Here's how the part is built. I have some questions about the finished solid (model axes, mm). Round coordinates to 2 decimals unless told otherwise and drop trailing zeros. Loops run counter-clockwise (first coordinate to the right, second up) from the corner with the lowest first, then second, coordinate; pieces in that order, holes last. Notation, with made-up numbers: (-39.5, -9) - (-26.5, -9) arc R36 ccw to (-26.5, 27) - close; hole circle Ø8 at (31, 19.25). An arc over 180 degrees is marked (long way). Answer as a JSON object with one key per item and string values. Group by question number.
1) I want a section at B-B, the plane y = 0.6. Give the number of separate pieces and of enclosed holes in the cut face, then the cut area to 3 significant figures.
2) Will these pins go through, and if not, where does the flat tip stop? P1, Ø0.5, axis at y = 0.5, z = 80.5, coming from the +X side; P2, Ø0.5, axis at y = 0.5, z = -101.5, coming from the -X side.
3) I want a section at D-D, the plane z = 86.5. Please give me the cut outline in (x, y), then the cut area to 3 significant figures.
4) If we mould it in two halves opening along X, with no side actions, what happens to faces 1 (the face through (41.748, 0.493, 105.846)), 2 (the face through (33.07, 0.49, 104.63)), 3 (the face through (1, 0, -2))? For each: pulls with the +X half, pulls with the -X half, needs draft (parallel to the pull), parting line crosses it, or undercut.
5) If I drill on line 1 along Z through (x, y) = (-19, 0.3); line 2 along Z through (x, y) = (12.5, 0.8); line 3 along Z through (x, y) = (26.5, 0.5), over which ranges is the centre line in solid material (lowest first)? Write a range as [from, to].
6) I want a section at C-C, the plane z = 36.5. Please give me the cut outline in (x, y).
7) I want a section at A-A, the plane x = -24. Please give me the cut outline in (y, z).
from build123d import *

# Parameters (mm, degrees)
SKETCH1_R           = 1.95
BOSS_EXTRUDE1_DEPTH = 1


with BuildPart() as part:
    # Sketch1 → Boss-Extrude1 (new body)
    with BuildSketch(Plane(origin=(0, 0, 0), x_dir=(1, 0, 0), z_dir=(0, 1, 0))):
        with BuildLine():
            Line((-31.75, 116.06601718), (-12.75, 116.06601718))
            Line((-12.75, 116.06601718), (-12.75, 96.06601718))
            Line((-12.75, 96.06601718), (-11.75, 96.06601718))
            Line((-11.75, 96.06601718), (11.75, 96.06601718))
            Line((11.75, 96.06601718), (12.75, 96.06601718))
            Line((12.75, 96.06601718), (12.75, 116.06601718))
            Line((12.75, 116.06601718), (31.75, 116.06601718))
            ThreePointArc((31.75, 116.06601718), (41.75, 106.06601718), (31.75, 96.06601718))
            Line((31.75, 96.06601718), (31.75, 81.06601718))
            Line((31.75, 81.06601718), (11.75, 81.06601718))
            Line((11.75, 81.06601718), (11.75, 80.06601718))
            Line((11.75, 80.06601718), (21.75, 80.06601718))
            Line((21.75, 80.06601718), (21.75, -80.06601718))
            Line((21.75, -80.06601718), (11.75, -80.06601718))
            Line((11.75, -80.06601718), (11.75, -81.06601718))
            Line((11.75, -81.06601718), (31.75, -81.06601718))
            Line((31.75, -81.06601718), (31.75, -96.06601718))
            ThreePointArc((31.75, -96.06601718), (41.75, -106.06601718), (31.75, -116.06601718))
            Line((31.75, -116.06601718), (12.75, -116.06601718))
            Line((12.75, -116.06601718), (12.75, -96.06601718))
            Line((12.75, -96.06601718), (11.75, -96.06601718))
            Line((11.75, -96.06601718), (-11.75, -96.06601718))
            Line((-11.75, -96.06601718), (-12.75, -96.06601718))
            Line((-12.75, -96.06601718), (-12.75, -116.06601718))
            Line((-12.75, -116.06601718), (-31.75, -116.06601718))
            ThreePointArc((-31.75, -116.06601718), (-41.75, -106.06601718), (-31.75, -96.06601718))
            Line((-31.75, -96.06601718), (-31.75, -81.06601718))
            Line((-31.75, -81.06601718), (-11.75, -81.06601718))
            Line((-11.75, -81.06601718), (-11.75, -80.06601718))
            Line((-11.75, -80.06601718), (-21.75, -80.06601718))
            Line((-21.75, -80.06601718), (-21.75, 80.06601718))
            Line((-21.75, 80.06601718), (-11.75, 80.06601718))
            Line((-11.75, 80.06601718), (-11.75, 81.06601718))
            Line((-11.75, 81.06601718), (-31.75, 81.06601718))
            Line((-31.75, 81.06601718), (-31.75, 96.06601718))
            ThreePointArc((-31.75, 96.06601718), (-41.75, 106.06601718), (-31.75, 116.06601718))
        make_face()
        with Locations(Location((-31.75, 106.06601718, 0), (0, 0, 270))):
            Circle(SKETCH1_R, mode=Mode.SUBTRACT)
        with Locations(Location((31.75, 106.06601718, 0), (0, 0, 90))):
            Circle(SKETCH1_R, mode=Mode.SUBTRACT)
        with Locations(Location((31.75, -106.06601718, 0), (0, 0, 270))):
            Circle(SKETCH1_R, mode=Mode.SUBTRACT)
        with Locations(Location((-31.75, -106.06601718, 0), (0, 0, 90))):
            Circle(SKETCH1_R, mode=Mode.SUBTRACT)
    extrude(amount=BOSS_EXTRUDE1_DEPTH)


solid = part.part
Outcome:
{
 "1": {"separate pieces": "1", "enclosed holes": "4", "area": "11,000 mm^2"},
 "2": {"P1": "x = 11.75", "P2": "x = -40.77"},
 "3": {"outline": "(-31.75, 0) - (31.75, 0) - (31.75, 1) - (-31.75, 1) - close", "area": "63.5 mm^2"},
 "4": {"face 1": "pulls with the +X half", "face 2": "undercut", "face 3": "needs draft"},
 "5": {"line 1": "[-116.07, -81.07], [-80.07, 80.07], [81.07, 116.07]", "line 2": "[-96.07, -81.07], [-80.07, 80.07], [81.07, 96.07]", "line 3": "[-116.07, -81.07], [81.07, 116.07]"},
 "6": {"outline": "(-21.75, 0) - (21.75, 0) - (21.75, 1) - (-21.75, 1) - close"},
 "7": {"outline": "(0, -116.07) - (1, -116.07) - (1, -81.07) - (0, -81.07) - close; (0, 81.07) - (1, 81.07) - (1, 116.07) - (0, 116.07) - close"}
}
